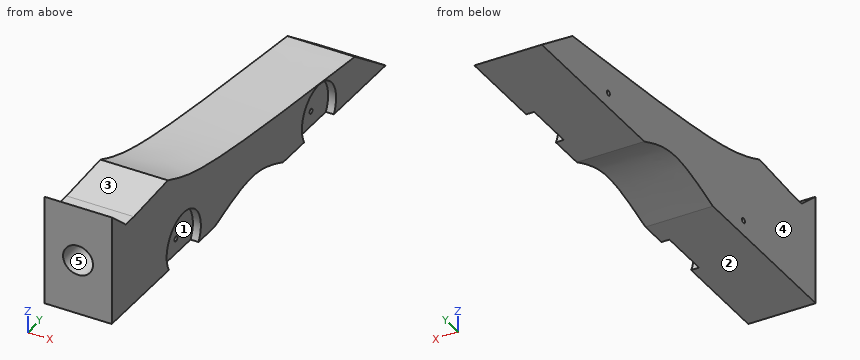
```python
from build123d import *

# Parameters (mm, degrees)
F1_DEPTH = 21.43125
F2_R     = 9.525
F3_DEPTH = 50.8
F4_R     = 1.5875
F6_DEPTH = 43.18
F7_R     = 19.05
F8_DEPTH = 5.08


with BuildPart() as f1:
    # F0 (on Right) → F1 (new body, symmetric)
    with BuildSketch(Plane.YZ):
        Polygon((-152.4, 69.85), (-152.4, 0), (152.4, 0), (152.4, 19.05), align=None)
    extrude(amount=F1_DEPTH, both=True)

    # F2 (on face) → F3 (cut)
    with BuildSketch(Plane.XZ.offset(152.4)):
        with Locations((0, 34.925)):
            Circle(F2_R)
    extrude(amount=-F3_DEPTH, mode=Mode.SUBTRACT)

    # F4 (on face) → F6 (intersect)
    with BuildSketch(Plane.YZ.offset(21.43125)):
        with BuildLine():
            Line((152.4, 0), (118.0612299003, 24.77312835))
            add(Edge.make_bspline(
                [(-89.9518863056, 59.4419810509), (-78.3312719762, 54.2757015098), (-46.7012859115, 40.2136781728), (104.83454077, 26.4256487446), (118.0612299003, 24.77312835)],
                knots=[0, 0, 0, 0, 0.3407661179, 0.9275264848, 0.9275264848, 0.9275264848, 0.9275264848], degree=3))
            Line((-89.9518863056, 59.4419810509), (-127.7775764465, 56.6512197256))
            Line((-127.7775764465, 56.6512197256), (-136.9280835145, 56.6512197256))
            Line((-136.9280835145, 56.6512197256), (-152.4, 69.85))
            Line((-152.4, 69.85), (-152.4, 0))
            Line((-152.4, 0), (-37.9903614521, 0))
            add(Edge.make_bspline(
                [(-37.9903614521, 0), (-22.7117503508, 5.0129187767), (5.7637416088, 14.3557397552), (27.9814406153, 4.5462011009), (38.2781662047, 0)],
                knots=[0, 0, 0, 0, 0.5365530163, 1, 1, 1, 1], degree=3))
            Line((38.2781662047, 0), (152.4, 0))
        make_face()
        with Locations((-72.0704272389, 9.525)):
            Circle(F4_R, mode=Mode.SUBTRACT)
        with Locations((78.2117620111, 9.525)):
            Circle(F4_R, mode=Mode.SUBTRACT)
    extrude(amount=-F6_DEPTH, mode=Mode.INTERSECT)

    # F7 (on face) → F8 (cut)
    with BuildSketch(Plane.YZ.offset(21.43125)):
        with Locations((-72.2883281696, 9.525)):
            Circle(F7_R)
        with Locations((78.2117247581, 9.5152128488)):
            Circle(F7_R)
    extrude(amount=-F8_DEPTH, mode=Mode.SUBTRACT)


solid = f1.part
```
Work out the finished part from the listing and answer in its coordinate system (mm). Face numbers are marked on the shaded views. A direction names the side the tool comes from. Round coordinates to 2 decimals unless told otherwise and drop trailing zeros. Loops run counter-clockwise (first coordinate to the right, second up) from the corner with the lowest first, then second, coordinate; pieces in that order, holes last. Notation, with made-up numbers: (-27.5, -40) -> (18.5, -40) arc R18 ccw to (18.5, -30) -> close; hole circle Ø3 at (7.5, 37). An arc over 180 degrees is marked (long way). Write each question's results on one line, items separated by ' | '. Start each with the question number.
1. A tool of negligible diameter and unlimited length cuts with its end or side. For the marked faces 1 and 2, from which of +Z, -Z, +X, -X, +Y, -Y can it reach the whole face along a straight path? Write none if from no direction.
2. Given pin 1 Ø2.5 at (x, y) = (-9, -133.5) entering from +Z; pin 2 Ø14.5 at (y, z) = (86, 17) entering from +X; pin 3 Ø5 at (x, y) = (9.5, -88.5) entering from +Z, each flat-ended and moving along its own axis, determine where each tip first touches the part or whether it passes through.
3. Find the intervals of material crossed by probe 1 along Z at (x, y) = (8.5, 79); probe 2 along Z at (x, y) = (-14, -47); probe 3 along Z at (x, y) = (-1, -118), in increasing order. Write a range as from..to.
4. For a pull along X with two mould halves and no side action, classify the marked faces 3, 4 and 5 as +X half, -X half, draft (parallel to the pull), parting line (faces both ways), or undercut.
5. Section B-B (x = -17) is taken. State how many separate pieces and enclosed holes the cut face has, plus the area to 3 significant figures.
6. Section C-C (z = 15.5) is taken. Determine the outline of the cut face in (x, y), plus the area to 3 significant figures.
Evaluation:
1) face 1: +X | face 2: -Z, +X, -X, +Y, -Y
2) pin 1: stops at z = 56.65 | pin 2: stops at x = 16.35 | pin 3: stops at z = 59.44
3) probe 1: z = 0..8.15, 10.9..28.85 | probe 2: z = 0..45.57 | probe 3: z = 0..25.45, 44.4..57.37
4) face 3: draft | face 4: -X half | face 5: undercut
5) separate pieces: 1 | enclosed holes: 2 | area: 11,500 mm2
6) outline: (-21.43, -152.4) -> (21.43, -152.4) -> (21.43, -90.38) -> (16.35, -90.38) -> (16.35, -54.2) -> (21.43, -54.2) -> (21.43, 60.13) -> (16.35, 60.13) -> (16.35, 96.3) -> (21.43, 96.3) -> (21.43, 130.91) -> (-21.43, 130.91) -> close | area: 11,800 mm2
